Geometry check sheet. Reference: the model listing, model coordinates, mm. A direction names the side the tool comes from. Give positions to 0.01 mm unless a question says otherwise; leave off trailing zeros. Loops run counter-clockwise (first coordinate to the right, second up) from the corner with the lowest first, then second, coordinate; pieces in that order, holes last.
1. Tool access check on faces 1 (the flat face through (0, -2, -2)), 2 (the flat face through (2, 14, 7.036)), 3 (the flat face through (2, -5.461, 11)), 4 (the flat face through (2, -33, 2.035)). Record the directions out of +Z, -Z, +X, -X, +Y, -Y that give a thin tool (end or side, any length) a straight path to the whole face; none if there is none.
2. Cross-section at D-D, the plane z = -1. Record the cut outline in (x, y).
3. Cross-section at A-A, the plane z = 10.75. Record the cut outline in (x, y).
4. Cross-section at B-B, the plane x = 1.15. Record the cut outline in (y, z), plus the area to 3 significant figures.
5. Material ranges on L1, parallel to Y at x = 0.8, z = 9; L2, parallel to Z at x = 1.35, y = -31; L3, parallel to Z at x = 3.05, y = -27.5, recorded low to high.
6. Release check for a two-part mould opening along Z. For faces 5 (the flat face through (2, -30.536, -3)), 6 (the flat face through (2, 0, 15.036)), 7 (the flat face through (2, 33.464, 6)) record: +Z half, -Z half, draft (parallel to the pull), parting line (faces both ways), or undercut.
7. Go/stop test with flat-tipped pins: pin 1 Ø1.5 at (x, z) = (4, -7.5) entering from -Y; pin 2 Ø2.5 at (x, y) = (3, 11) entering from +Z; pin 3 Ø3 at (x, z) = (1.5, -5) entering from +Y; pin 4 Ø2.5 at (x, z) = (2.5, 10.5) entering from -Y. Record where each tip stops, or that it passes through.
8. Cross-section at C-C, the plane y = 6. Record the cut outline in (x, z).
Autodesk Inventor part; units mm, degrees
ref_plane "YZ Plane" through (0, 0, 0) normal (1, 0, 0) x (0, 1, 0)
ref_plane "XZ Plane" through (0, 0, 0) normal (0, 1, 0) x (-1, 0, 0)
ref_plane "XY Plane" through (0, 0, 0) normal (0, 0, 1) x (1, 0, 0)
sketch "dds" plane through (0, -35.5355, 2.0355) normal (1, 0, 0) x (0, 1, 0)
  line L0 (0, -9.9999) -> (5, -9.9999)
  line L1 (0, -9.9999) -> (0, -15)
  line L2 (0, -15) -> (5, -15)
  line L3 (0, 0) -> (5, 0)
  line L4 (5, -9.9999) -> (5, 0)
  line L5 (5, -15) -> (59, -15)
  line L6 (0, 0) -> (0, 5)
  line L7 (69, 5) -> (69, 13)
  line L8 (69, 5) -> (69, -5)
  arc A0 (59, -15) -> (69, -5) centre (59, -5) ccw
  line L9 (69, 13) -> (58.8965, 13)
  line L10 (58.8965, 13) -> (58.8965, 5)
  line L11 (40.1783, 13) -> (30.0747, 13)
  line L12 (40.1783, 5) -> (40.1783, 13)
  line L13 (30.0747, 13) -> (30.0747, 5)
  line L14 (0, 5) -> (30.0747, 5)
  line L15 (40.1783, 5) -> (58.8965, 5)
  point P0 (69, -15)
  point P1 (8.1162, -2.0146)
  dimension "d0" = 10
  dimension "d1" = 8
extrude "Side" add sketch "dds" along normal blind 5
properties part number "Side"
Result:
1. face 1: +Z, -Z, -X, +Y, -Y
1. face 2: +Z, +X, -X
1. face 3: +Z, +X, -X, -Y
1. face 4: +X, -X, -Y
2. outline: (0, -30.54) - (5, -30.54) - (5, 33.46) - (0, 33.46) - close
3. outline: (0, -5.46) - (5, -5.46) - (5, 4.64) - (0, 4.64) - close; (0, 23.36) - (5, 23.36) - (5, 33.46) - (0, 33.46) - close
4. outline: (-35.54, -12.96) - (23.46, -12.96) arc R10 ccw to (33.46, -2.96) - (33.46, 15.04) - (23.36, 15.04) - (23.36, 7.04) - (4.64, 7.04) - (4.64, 15.04) - (-5.46, 15.04) - (-5.46, 7.04) - (-35.54, 7.04) - (-35.54, 2.04) - (-30.54, 2.04) - (-30.54, -7.96) - (-35.54, -7.96) - close
4. area: 1,470 mm2
5. L1: y = -5.46 to 4.64, 23.36 to 33.46
5. L2: z = -12.96 to -7.96, 2.04 to 7.04
5. L3: z = -12.96 to 7.04
6. face 5: undercut
6. face 6: +Z half
6. face 7: draft
7. pin 1: stops at y = -35.54
7. pin 2: stops at z = 7.04
7. pin 3: stops at y = 33.45
7. pin 4: stops at y = -5.46
8. outline: (0, -12.96) - (5, -12.96) - (5, 7.04) - (0, 7.04) - close
